Geometry check sheet. Reference: drawing and pictorial views, mm from the part's lowest x, y, z. A direction names the side the tool comes from. Give positions to 0.01 mm unless a question says otherwise; leave off trailing zeros. Loops run counter-clockwise (first coordinate to the right, second up) from the corner with the lowest first, then second, coordinate; pieces in that order, holes last. Notation, with made-up numbers: (-10.5, -3.5) -> (12.5, -3.5) arc R12 ccw to (12.5, 2.5) -> close; hole circle Ø2 at (24.5, -27). An arc over 180 degrees is marked (long way). Write each question's results on one line, items separated by ' | '. Start each with the question number.
1. Cross-section at B-B on x = 37.5. Record the boundary of the cut face in (y, z), and give its area (3 significant figures).
2. Cross-section at C-C on z = 6.5. Record the boundary of the cut face in (x, y) (3 decimals).
3. Cross-section at D-D on x = 55. Record the boundary of the cut face in (y, z), and give its area (3 significant figures).
4. Gauge pin test, flat ends, axial feed: pin 1 Ø3 at (y, z) = (98.5, 8.5) entering from +X; pin 2 Ø1 at (x, z) = (28, 5) entering from -Y (3 decimals); pin 3 Ø4 at (x, y) = (87.5, 67.5) entering from -Z. Record the tip position at first contact, or that the pin passes through.
5. Tool access check on the marked faces 1 and 2. Record the directions out of +Z, -Z, +X, -X, +Y, -Y that give a thin tool (end or side, any length) a straight path to the whole face; none if there is none.
6. Cross-section at A-A on y = 55. Record the boundary of the cut face in (x, z).
7. Material ranges on L1, parallel to X at y = 39.5, z = 2.5 (1 decimal); L2, parallel to Y at x = 72.25, z = 4.75; L3, parallel to Z at x = 80, y = 63.5, recorded low to high. Write a range as from..to.
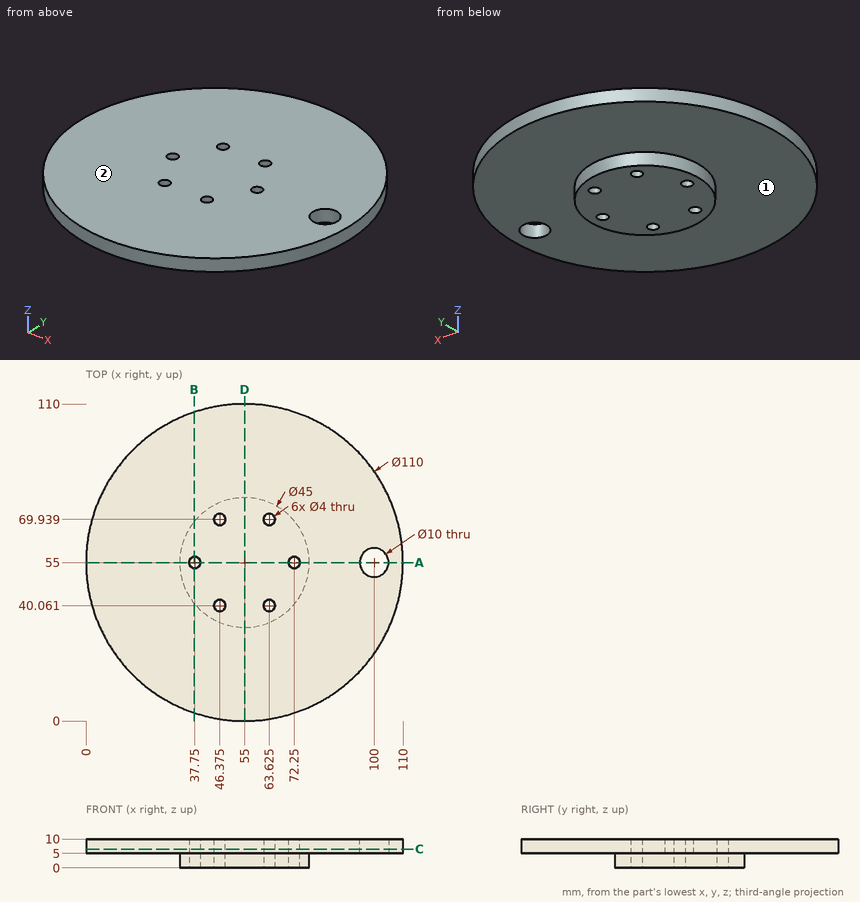
Geometry says:
1) outline: (2.86, 5) -> (40.86, 5) -> (40.86, 0) -> (53.02, 0) -> (53.02, 10) -> (2.86, 10) -> close; (56.98, 0) -> (69.14, 0) -> (69.14, 5) -> (107.14, 5) -> (107.14, 10) -> (56.98, 10) -> close | area: 623 mm^2
2) outline: circle Ø110 at (55, 55); hole circle Ø4 at (37.75, 55); hole circle Ø4 at (46.375, 40.061); hole circle Ø4 at (46.375, 69.939); hole circle Ø4 at (63.625, 40.061); hole circle Ø4 at (63.625, 69.939); hole circle Ø4 at (72.25, 55); hole circle Ø10 at (100, 55)
3) outline: (0, 5) -> (32.5, 5) -> (32.5, 0) -> (77.5, 0) -> (77.5, 5) -> (110, 5) -> (110, 10) -> (0, 10) -> close | area: 775 mm^2
4) pin 1: x = 90.51 | pin 2: y = 6.805 | pin 3: z = 5
5) face 1: -Z | face 2: +Z, +X, -X, +Y, -Y
6) outline: (0, 5) -> (32.5, 5) -> (32.5, 0) -> (35.75, 0) -> (35.75, 10) -> (0, 10) -> close; (39.75, 0) -> (70.25, 0) -> (70.25, 10) -> (39.75, 10) -> close; (74.25, 0) -> (77.5, 0) -> (77.5, 5) -> (95, 5) -> (95, 10) -> (74.25, 10) -> close; (105, 5) -> (110, 5) -> (110, 10) -> (105, 10) -> close
7) L1: 38.7..44.5, 48.3..61.7, 65.5..71.3 | L2: 40.55..53, 57..69.45 | L3: 5..10
